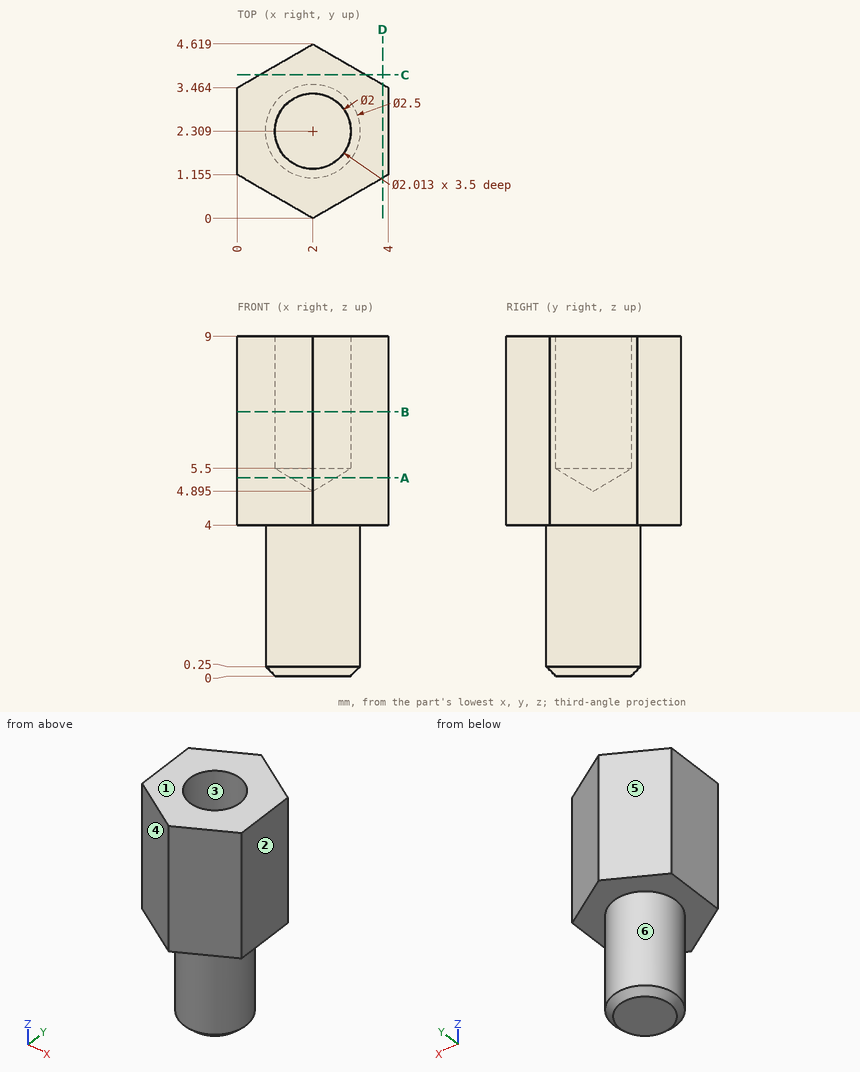
Could you check a few things on this drawing? It's one solid part, dimensions in mm from its lowest x, y, z. A direction names the side the tool comes from. Coordinates: 2 decimals unless noted, no trailing zeros. Write each loop counter-clockwise with the first axis right and the second up, starting at its lowest first coordinate (ties: lowest second). Pieces come first, ordered by that corner, then holes. Notation, with made-up numbers: M 42.5,68.25 L 75.5,68.25 A30 cw 75.5,90.25 Z; hole C 42.5,-16.75 d7. An arc over 180 degrees is marked long. One line per question, with ' | ' between items.
1) Imagine slicing it at D-D, the plane x = 3.85. Write out the boundary of the cut face in (y, z).
Checks:
outline: M 1.07,4 L 3.55,4 L 3.55,9 L 1.07,9 Z
2) For pin 1 Ø1 at (x, z) = (2.5, 2) entering from -Y; pin 2 Ø1.8 at (x, y) = (2, 2.31) entering from +Z, each with a flat end and sliding along its axis, tell me the tip position at first contact or that it passes through.
Checks:
pin 1: y = 1.06 | pin 2: z = 5.44
3) If we mould it in two halves opening along X, with no side actions, what happens to the marked faces 1, 2, 3 and 4? For each: released by +X, released by -X, zero draft, split by the parting line, or undercut.
Checks:
face 1: zero draft | face 2: released by +X | face 3: undercut | face 4: released by -X
4) Imagine slicing it at B-B, the plane z = 7. Write out the boundary of the cut face in (x, y) (1 decimal).
Checks:
outline: M 0,1.2 L 2,0 L 4,1.2 L 4,3.5 L 2,4.6 L 0,3.5 Z; hole C 2,2.3 d2
5) For the marked faces 5 and 6, which set-ups out of +Z, -Z, +X, -X, +Y, -Y let a thin tool reach every point of the face, with its end or its side?
Checks:
face 5: +Z, -Z, -X, +Y | face 6: -Z
6) Imagine slicing it at A-A, the plane z = 5.25. Write out the boundary of the cut face in (x, y) (1 decimal).
Checks:
outline: M 0,1.2 L 2,0 L 4,1.2 L 4,3.5 L 2,4.6 L 0,3.5 Z; hole C 2,2.3 d1.2
7) Imagine slicing it at C-C, the plane y = 3.8. Write out the boundary of the cut face in (x, z), and give its area (3 significant figures).
Checks:
outline: M 0.58,4 L 3.42,4 L 3.42,9 L 0.58,9 Z | area: 14.2 mm²
8) I need wall thicknesses on probe 1 along X at (y, z) = (2.45, 8); probe 2 along Z at (x, y) = (1.8, 4.15); probe 3 along Y at (x, z) = (1.75, 8.75) (1 decimal). Which ranges of each line are inside material? Lowest first, please. Write a range as [from, to].
Checks:
probe 1: [0, 1], [3, 4] | probe 2: [4, 9] | probe 3: [0.1, 1.3], [3.3, 4.5]
